```python
from build123d import *

# Parameters (mm, degrees)
SKETCH1_R                = 20
BOSS_EXTRUDE1_DEPTH      = 65
BOSS_EXTRUDE2_DEPTH      = 3
BOSS_EXTRUDE2_DEPTH_BACK = 68
SKETCH2_R                = 7.5
BOSS_EXTRUDE3_DEPTH      = 90
BOSS_EXTRUDE3_DEPTH_BACK = 10
SKETCH3_R                = 1.5


with BuildPart() as part:
    # Sketch1 → Boss-Extrude1 (new body)
    with BuildSketch(Plane(origin=(0, 0, 0), x_dir=(1, 0, 0), z_dir=(0, 1, 0))):
        with Locations(Location((0, 0, 0), (0, 0, 270))):
            Circle(SKETCH1_R)
    extrude(amount=BOSS_EXTRUDE1_DEPTH)

    # Sketch2 → Boss-Extrude2 (add, two sides: drawn at the far end of the back side and taken through both)
    with BuildSketch(Plane(origin=(0, 65, 0), x_dir=(1, 0, 0), z_dir=(0, 1, 0)).offset(-BOSS_EXTRUDE2_DEPTH_BACK)):
        with Locations(Location((0, 0, 0), (0, 0, 270))):
            Circle(SKETCH2_R)
    extrude(amount=BOSS_EXTRUDE2_DEPTH + BOSS_EXTRUDE2_DEPTH_BACK)

    # Sketch3 → Boss-Extrude3 (add, two sides: drawn at the far end of the back side and taken through both)
    with BuildSketch(Plane(origin=(0, 0, 0), x_dir=(1, 0, 0), z_dir=(0, 1, 0)).offset(-BOSS_EXTRUDE3_DEPTH_BACK)):
        with Locations(Location((0, 0, 0), (0, 0, 270))):
            Circle(SKETCH3_R)
    extrude(amount=BOSS_EXTRUDE3_DEPTH + BOSS_EXTRUDE3_DEPTH_BACK)


solid = part.part
```
The listing builds one solid part. Answer for the finished solid, in the listing's coordinates (mm). A direction names the side the tool comes from. Give positions to 0.01 mm unless a question says otherwise; leave off trailing zeros. Loops run counter-clockwise (first coordinate to the right, second up) from the corner with the lowest first, then second, coordinate; pieces in that order, holes last. Notation, with made-up numbers: M 6,5.5 L 63,5.5 A20 ccw 63,20.5 Z; hole C -5.5,18 d6. An arc over 180 degrees is marked long. One line per item, written item: value.
1. Each of these flat-tipped pins is pushed along its axis until it touches: P1, Ø8, axis at y = 24.5, z = -5, coming from the -X side (3 decimals); P2, Ø3, axis at y = 7, z = 9, coming from the +X side; P3, Ø10, axis at y = 28.5, z = 15, coming from the -X side. Where does it stop, or does it pass through?
Found:
P1: x = -19.975
P2: x = 18.54
P3: x = -17.32
2. Section C-C on y = 30 is taken. Determine the outline of the cut face in (x, z), plus the area to 3 significant figures.
Found:
outline: C 0,0 d40
area: 1,260 mm^2
3. For faces 1 (the face through (0, -10, 0)), 2 (the face through (0, 0, 9)), 3 (the face through (0, 65, 9)), determine the directions among +Z, -Z, +X, -X, +Y, -Y from which every point of the face is accessible in a straight line to the end or side of a thin tool.
Found:
face 1: +Z, -Z, +X, -X, -Y
face 2: -Y
face 3: +Y
4. Section D-D on x = 12 is taken. Determine the outline of the cut face in (y, z), plus the area to 3 significant figures.
Found:
outline: M 0,-16 L 65,-16 L 65,16 L 0,16 Z
area: 2,080 mm^2
5. Section A-A on x = 0 is taken. Determine the outline of the cut face in (y, z).
Found:
outline: M -10,-1.5 L -3,-1.5 L -3,-7.5 L 0,-7.5 L 0,-20 L 65,-20 L 65,-7.5 L 68,-7.5 L 68,-1.5 L 90,-1.5 L 90,1.5 L 68,1.5 L 68,7.5 L 65,7.5 L 65,20 L 0,20 L 0,7.5 L -3,7.5 L -3,1.5 L -10,1.5 Z
6. Section B-B on z = 0 is taken. Determine the outline of the cut face in (x, y).
Found:
outline: M -20,0 L -7.5,0 L -7.5,-3 L -1.5,-3 L -1.5,-10 L 1.5,-10 L 1.5,-3 L 7.5,-3 L 7.5,0 L 20,0 L 20,65 L 7.5,65 L 7.5,68 L 1.5,68 L 1.5,90 L -1.5,90 L -1.5,68 L -7.5,68 L -7.5,65 L -20,65 Z
7. Find the intervals of material crossed by probe 1 along Y at (x, z) = (-12, 6.5); probe 2 along X at (y, z) = (11, -0.5); probe 3 along Z at (x, y) = (5, 41), in increasing order.
Found:
probe 1: 0 to 65
probe 2: -19.99 to 19.99
probe 3: -19.36 to 19.36
